Check sheet for the modelled part. Datum: model origin and axes. Units: mm. A direction names the side the tool comes from. Give positions to 0.01 mm unless a question says otherwise; leave off trailing zeros. Loops run counter-clockwise (first coordinate to the right, second up) from the corner with the lowest first, then second, coordinate; pieces in that order, holes last.
```python
from build123d import *

# Parameters (mm, degrees)
SKETCH_4_W           = 60
SKETCH_4_H           = 40
EXTRUDE_2_DEPTH      = 45
SKETCH_5_W           = 34
SKETCH_5_H           = 35
CUT_EXTRUDE_2_DEPTH  = 78.620873481
F_3_0MM_1_D          = 3
F_3_0MM_1_DEPTH      = 6
F_3_0MM_1_TIP        = 0.901290929
CUT_EXTRUDE_3_DEPTH  = 7.3
SKETCH_9_R           = 7
CUT_EXTRUDE_4_DEPTH  = 8.3
SKETCH_10_R          = 2.550838559
CUT_EXTRUDE_5_DEPTH  = 8.3
SKETCH_11_R          = 5
CUT_EXTRUDE_6_DEPTH  = 2
CUT_EXTRUDE_7_DEPTH  = 3
SKETCH_14_W          = 52.283643435
SKETCH_14_H          = 5.439682323
CUT_EXTRUDE_8_DEPTH  = 3
SKETCH_15_R          = 5
EXTRUDE_3_DEPTH      = 10
FILLET_1_R           = 10
F_3_0MM_2_D          = 3
SKETCH_18_R          = 2
CUT_EXTRUDE_9_DEPTH  = 8
CUT_EXTRUDE_10_DEPTH = 10
FILLET_2_R           = 10


with BuildPart() as part:
    # 草图4 → 凸台-拉伸2 (new body)
    with BuildSketch(Plane(origin=(0, 0, 0), x_dir=(1, 0, 0), z_dir=(0, 1, 0))):
        Rectangle(SKETCH_4_W, SKETCH_4_H)
    extrude(amount=EXTRUDE_2_DEPTH)

    # 草图5 → 切除-拉伸2 (cut, through all)
    with BuildSketch(Plane(origin=(30, 0, 0), x_dir=(0, 0, -1), z_dir=(1, 0, 0))):
        with Locations((3, 17.5)):
            Rectangle(SKETCH_5_W, SKETCH_5_H)
    extrude(amount=-CUT_EXTRUDE_2_DEPTH, mode=Mode.SUBTRACT)

    # Ø3.0mm 暗销孔1
    with Locations(Plane.XZ.offset(-35)):
        with Locations((24.25, -2.063956798), (-24.25, 7.936043202), (-24.25, -2.063956798), (24.25, 7.936043202)):
            Hole(F_3_0MM_1_D / 2, depth=F_3_0MM_1_DEPTH)
            with Locations((0, 0, -(F_3_0MM_1_DEPTH + F_3_0MM_1_TIP / 2))):  # 118° drill point
                Cone(0, F_3_0MM_1_D / 2, F_3_0MM_1_TIP, mode=Mode.SUBTRACT)

    # 草图8 → 切除-拉伸3 (cut)
    with BuildSketch(Plane.XZ.offset(-35)):
        Polygon((-20, -2.063956798), (-20, 14), (20, 14), (20, -8.063956798), (-20, -8.063956798), align=None)
    extrude(amount=-CUT_EXTRUDE_3_DEPTH, mode=Mode.SUBTRACT)

    # 草图9 → 切除-拉伸4 (cut)
    with BuildSketch(Plane.XZ.offset(-42.3)):
        with Locations(Location((10.009015473, 4.047123648, 0), (0, 0, 270))):
            Circle(SKETCH_9_R)
    extrude(amount=-CUT_EXTRUDE_4_DEPTH, mode=Mode.SUBTRACT)

    # 草图10 → 切除-拉伸5 (cut)
    with BuildSketch(Plane.XZ.offset(-42.3)):
        with Locations(Location((-10.440145967, 4.047123648, 0), (0, 0, 270))):
            Circle(SKETCH_10_R)
    extrude(amount=-CUT_EXTRUDE_5_DEPTH, mode=Mode.SUBTRACT)

    # 草图11 → 切除-拉伸6 (cut)
    with BuildSketch(Plane.XZ.offset(-42.3)):
        with Locations(Location((-10.440145967, 4.047123648, 0), (0, 0, 270))):
            Circle(SKETCH_11_R)
    extrude(amount=-CUT_EXTRUDE_6_DEPTH, mode=Mode.SUBTRACT)

    # 草图13 → 切除-拉伸7 (cut)
    with BuildSketch(Plane.XZ.offset(-35)):
        Polygon((-20, 4.395263317), (-27, 4.395263317), (-27, 2.895263317), (-20, 2.968021601), align=None)
        Polygon((20, 2.968021601), (20, 4.395263317), (27, 4.395263317), (27, 2.895263317), align=None)
    extrude(amount=-CUT_EXTRUDE_7_DEPTH, mode=Mode.SUBTRACT)

    # 草图14 → 切除-拉伸8 (cut)
    with BuildSketch(Plane(origin=(0, 0, 14), x_dir=(-1, 0, 0), z_dir=(0, 0, -1))):
        with Locations((0.858178282, 6.724921265)):
            Rectangle(SKETCH_14_W, SKETCH_14_H)
    extrude(amount=-CUT_EXTRUDE_8_DEPTH, mode=Mode.SUBTRACT)

    # 草图15 → 凸台-拉伸3 (add)
    with BuildSketch(Plane.XY.offset(20)):
        with Locations(Location((0, 22.5, 0), (0, 0, 180))):
            Circle(SKETCH_15_R)
        with BuildLine():
            Line((2, 24), (2, 21))
            ThreePointArc((2, 21), (-2.5, 22.5), (2, 24))
        make_face(mode=Mode.SUBTRACT)
    extrude(amount=EXTRUDE_3_DEPTH)

    # 圆角1
    fillet_1_edges = [part.edges().sort_by_distance(p)[0] for p in [
        (5, 22.5, 20),
    ]]
    fillet(fillet_1_edges, radius=FILLET_1_R - 0.0001)  # a hair under: the kernel refuses the full size

    # Ø3.0mm 暗销孔2 (through all)
    with Locations(Plane.XZ.offset(-35)):
        with Locations((15, -14.031978399), (-15, -14.031978399)):
            Hole(F_3_0MM_2_D / 2)

    # 草图18 → 切除-拉伸9 (cut)
    with BuildSketch(Plane(origin=(0, 45, 0), x_dir=(1, 0, 0), z_dir=(0, 1, 0))):
        with Locations(Location((-27.03202133, -14, 0), (0, 0, 270))):
            Circle(SKETCH_18_R)
        with Locations(Location((27.03202133, -14, 0), (0, 0, 90))):
            Circle(SKETCH_18_R)
    extrude(amount=-CUT_EXTRUDE_9_DEPTH, mode=Mode.SUBTRACT)

    # 草图20 → 切除-拉伸10 (cut)
    with BuildSketch(Plane.XZ.offset(-35)):
        with BuildLine():
            Line((-30, -7.5), (-30, -20))
            Line((-30, -20), (-17.5, -20))
            ThreePointArc((-17.5, -20), (-21.161165235, -11.161165235), (-30, -7.5))
        make_face()
        with BuildLine():
            Line((30, -20), (17.5, -20))
            ThreePointArc((17.5, -20), (21.161165235, -11.161165235), (30, -7.5))
            Line((30, -7.5), (30, -20))
        make_face()
    extrude(amount=-CUT_EXTRUDE_10_DEPTH, mode=Mode.SUBTRACT)

    # 圆角2
    fillet_2_edges = [part.edges().sort_by_distance(p)[0] for p in [
        (-17.5, 40, -20),
        (-30, 40, -7.5),
        (30, 40, -7.5),
        (17.5, 40, -20),
    ]]
    fillet(fillet_2_edges, radius=FILLET_2_R)


solid = part.part
```
(1) Release check for a two-part mould opening along Y. For faces 5 (the face through (0, 42.3, 3)), 6 (the face through (0, 7, 17)), 7 (the face through (0, 7, 20)) record: pulls with the +Y half, pulls with the -Y half, needs draft (parallel to the pull), parting line crosses it, or undercut.
(2) Section check D-D on z = -6.5. Record the boundary of the cut face in (x, y).
(3) Gauge pin test, flat ends, axial feed: pin 1 Ø12 at (x, y) = (8.5, 36) entering from +Z; pin 2 Ø10 at (x, z) = (-14.5, 2.5) entering from -Y; pin 3 Ø1 at (x, y) = (1, 35) entering from +Z. Record the tip position at first contact, or that the pin passes through.
(4) Access from +Z, -Z, +X, -X, +Y, -Y to the whole of each face (thin tool, end or side, straight path). Record for faces 1 (the face through (16.106, 40.07, -13.018)), 2 (the face through (25.05, 41.06, 14.26)), 3 (the face through (0, 9.445, 15)), 4 (the face through (27, 36, 4)).
(5) Section check A-A on z = 15. Record the boundary of the cut face in (x, y), plus the area to 3 significant figures.
(6) Material ranges on line 1 (Z direction, x = -15, y = 38.75); line 2 (Z direction, x = 1, y = 38); line 3 (Z direction, x = 15, y = 43), recorded low to high.
Computed values:
1. face 5: pulls with the -Y half
1. face 6: undercut
1. face 7: needs draft
2. outline: (-27.46, 35) - (-20, 35) - (-20, 42.3) - (20, 42.3) - (20, 35) - (27.46, 35) - (27.46, 45) - (-27.46, 45) - close
3. pin 1: stops at z = 21.37
3. pin 2: stops at y = 42.3
3. pin 3: stops at z = 20.45
4. face 1: +Y, -Y
4. face 2: +Y
4. face 3: -Z
4. face 4: -Y
5. outline: (-30, 0) - (30, 0) - (30, 45) - (28.76, 45) - (28.76, 37) - (25.3, 37) - (25.3, 45) - (-25.3, 45) - (-25.3, 37) - (-28.76, 37) - (-28.76, 45) - (-30, 45) - close; hole (-27, 4.01) - (25.28, 4.01) - (25.28, 9.44) - (-27, 9.44) - close
5. area: 2,360 mm2
6. line 1: z = -18.57 to -15.53, -12.53 to -8.06, 14 to 20
6. line 2: z = -20 to -8.06, 14 to 20
6. line 3: z = -18.57 to -15.53, -12.53 to -0.86, 8.96 to 20
